```python
from build123d import *

# Parameters (mm, degrees)
BOSS_EXTRUDE1_DEPTH            = 2.54
F_3_16_0_1875_DIAMETER_HOLE1_D = 4.7625
CHAMFER1_SIZE                  = 2.54
CHAMFER2_SIZE                  = 0.2


with BuildPart() as part:
    # Sketch1 → Boss-Extrude1 (new body)
    with BuildSketch(Plane.XY):
        Polygon((0, 0), (0, 50.8), (-25.4, 50.8), (-25.4, 0), (-25.4, -25.4), (50.8, -25.4), (50.8, 0), align=None)
    extrude(amount=BOSS_EXTRUDE1_DEPTH)

    # 3/16 (0.1875) Diameter Hole1 (through all)
    with Locations(Plane.XY.offset(2.54)):
        with Locations((-12.7, 38.1), (-12.7, 12.7), (-12.7, -12.7), (12.7, -12.7), (38.1, -12.7)):
            Hole(F_3_16_0_1875_DIAMETER_HOLE1_D / 2)

    # Chamfer1
    chamfer1_edges = [part.edges().sort_by_distance(p)[0] for p in [
        (50.8, 0, 1.27),
        (50.8, -25.4, 1.27),
        (-25.4, -25.4, 1.27),
        (-25.4, 50.8, 1.27),
        (0, 50.8, 1.27),
        (0, 0, 1.27),
    ]]
    chamfer(chamfer1_edges, length=CHAMFER1_SIZE)

    # Chamfer2
    chamfer2_edges = [part.edges().sort_by_distance(p)[0] for p in [
        (40.48125, -12.7, 2.54),
        (40.48125, -12.7, 0),
        (15.08125, -12.7, 2.54),
        (15.08125, -12.7, 0),
        (-10.31875, -12.7, 2.54),
        (-10.31875, -12.7, 0),
        (-10.31875, 12.7, 2.54),
        (-10.31875, 12.7, 0),
        (-10.31875, 38.1, 2.54),
        (-10.31875, 38.1, 0),
    ]]
    chamfer(chamfer2_edges, length=CHAMFER2_SIZE)


solid = part.part
```
Geometry: final body of the model. Coordinates: model frame, mm. Coordinates: 2 decimals unless noted, no trailing zeros. Order: outer loops, then holes, each group sorted by start corner. A loop starts at its lowest first (then second) coordinate and runs counter-clockwise, first axis right, second up. Notation, with made-up numbers: (30.5, 48) - (87.5, 48) arc R28 cw to (87.5, 71) - close; hole circle Ø2 at (-33, 0.25). An arc over 180 degrees is marked (long way). Return JSON: item names as keys, results as strings. Group by question number.
1. Material intervals for line 1 along Y through (x, z) = (-12.7, 0.7); line 2 along Y through (x, z) = (12.7, 1.2); line 3 along X through (y, z) = (26, 0.6), sorted ascending. Write a range as [from, to].
2. Pin query (flat end, axial travel): pin 1 (0.8 mm diameter, centred on y = 27, z = 1.5, fed in from +X); pin 2 (4.5 mm diameter, centred on x = -12.7, y = 12.7, fed in from -Z). Return the tip coordinate at first contact, or that it passes through.
3. Cut plane B-B (z = 0.6). Output: boundary loops of the cut face in (x, y).
4. Pull-direction query (Y, two-part tool) for faces 1 (the face through (-12.39, 40.46, 1.26)), 2 (the face through (-25.4, 13, 1)), 3 (the face through (49.55, -1.29, 1.25)), 4 (the face through (-13.98, -10.69, 1.26)); classes: pulls with the +Y half, pulls with the -Y half, needs draft (parallel to the pull), parting line crosses it, or undercut.
5. Cut plane A-A (y = 12.7). Output: boundary loops of the cut face in (x, z).
6. Cut plane C-C (y = -12.7). Output: boundary loops of the cut face in (x, z), plus the area to 3 significant figures.
Resolved:
{
 "1": {"line 1": "y = [-25.4, -15.08], [-10.32, 10.32], [15.08, 35.72], [40.48, 50.8]", "line 2": "y = [-25.4, -15.08], [-10.32, 0]", "line 3": "x = [-25.4, 0]"},
 "2": {"pin 1": "stops at x = 0", "pin 2": "passes through"},
 "3": {"outline": "(-25.4, -22.86) - (-22.86, -25.4) - (48.26, -25.4) - (50.8, -22.86) - (50.8, -2.54) - (48.26, 0) - (2.54, 0) - (0, 2.54) - (0, 48.26) - (-2.54, 50.8) - (-22.86, 50.8) - (-25.4, 48.26) - close; hole circle Ø4.76 at (-12.7, -12.7); hole circle Ø4.76 at (-12.7, 12.7); hole circle Ø4.76 at (-12.7, 38.1); hole circle Ø4.76 at (12.7, -12.7); hole circle Ø4.76 at (38.1, -12.7)"},
 "4": {"face 1": "undercut", "face 2": "needs draft", "face 3": "pulls with the +Y half", "face 4": "undercut"},
 "5": {"outline": "(-25.4, 0) - (-15.28, 0) - (-15.08, 0.2) - (-15.08, 2.34) - (-15.28, 2.54) - (-25.4, 2.54) - close; (-10.32, 0.2) - (-10.12, 0) - (0, 0) - (0, 2.54) - (-10.12, 2.54) - (-10.32, 2.34) - close"},
 "6": {"outline": "(-25.4, 0) - (-15.28, 0) - (-15.08, 0.2) - (-15.08, 2.34) - (-15.28, 2.54) - (-25.4, 2.54) - close; (-10.32, 0.2) - (-10.12, 0) - (10.12, 0) - (10.32, 0.2) - (10.32, 2.34) - (10.12, 2.54) - (-10.12, 2.54) - (-10.32, 2.34) - close; (15.08, 0.2) - (15.28, 0) - (35.52, 0) - (35.72, 0.2) - (35.72, 2.34) - (35.52, 2.54) - (15.28, 2.54) - (15.08, 2.34) - close; (40.48, 0.2) - (40.68, 0) - (50.8, 0) - (50.8, 2.54) - (40.68, 2.54) - (40.48, 2.34) - close", "area": "157 mm²"}
}
